Here's how the part is built. I have some questions about the finished solid (model axes, mm). Face numbers are marked on the shaded views. A direction names the side the tool comes from. Give positions to 0.01 mm unless a question says otherwise; leave off trailing zeros. Loops run counter-clockwise (first coordinate to the right, second up) from the corner with the lowest first, then second, coordinate; pieces in that order, holes last.
Q1. Suppose I cut it at C-C (z = 7). List the corners of the cut face in (x, y) for me.
Q2. Suppose I cut it at D-D (x = 0). List the corners of the cut face in (y, z) for me, and give its area (3 significant figures).
Q3. Suppose I cut it at B-B (x = 5). List the corners of the cut face in (y, z) for me, and give its area (3 significant figures).
Q4. Thinking about a two-plate mould opening in Z: for the marked faces 3, 4 and 5, which applies, pulls with the +Z half, pulls with the -Z half, needs draft (parallel to the pull), parting line crosses it, or undercut?
Q5. Suppose I cut it at A-A (z = 2). List the corners of the cut face in (x, y) for me.
Q6. I need wall thicknesses on probe 1 along X at (y, z) = (27.05, 0); probe 2 along Z at (x, y) = (6, 15.25); probe 3 along Y at (x, z) = (-2.5, 4.75). Which ranges of each line are inside material? Lowest first, please.
Q7. For the marked faces 1 and 2, which set-ups out of +Z, -Z, +X, -X, +Y, -Y let a thin tool reach every point of the face, with its end or its side?
```python
from build123d import *

# Parameters (mm, degrees)
SKETCH1_W           = 22
SKETCH1_H           = 28
BOSS_EXTRUDE1_DEPTH = 5
SKETCH2_W           = 22
SKETCH2_H           = 5
BOSS_EXTRUDE2_DEPTH = 20
SKETCH3_W           = 22
SKETCH3_H           = 28
BOSS_EXTRUDE3_DEPTH = 5
SKETCH4_R           = 1.55
CUT_EXTRUDE1_DEPTH  = 30
SKETCH5_W           = 22
SKETCH5_H           = 20
CUT_EXTRUDE2_DEPTH  = 1.5
SKETCH6_W           = 22
SKETCH6_H           = 20
CUT_EXTRUDE3_DEPTH  = 1.5


with BuildPart() as part:
    # Sketch1 → Boss-Extrude1 (new body)
    with BuildSketch(Plane(origin=(0, 0, 0), x_dir=(1, 0, 0), z_dir=(0, 1, 0))):
        Rectangle(SKETCH1_W, SKETCH1_H)
    extrude(amount=BOSS_EXTRUDE1_DEPTH)

    # Sketch2 → Boss-Extrude2 (add)
    with BuildSketch(Plane(origin=(0, 5, 0), x_dir=(1, 0, 0), z_dir=(0, 1, 0))):
        with Locations((0, -11.5)):
            Rectangle(SKETCH2_W, SKETCH2_H)
        with Locations((0, 11.5)):
            Rectangle(SKETCH2_W, SKETCH2_H)
    extrude(amount=BOSS_EXTRUDE2_DEPTH)

    # Sketch3 → Boss-Extrude3 (add)
    with BuildSketch(Plane(origin=(0, 25, 0), x_dir=(1, 0, 0), z_dir=(0, 1, 0))):
        Rectangle(SKETCH3_W, SKETCH3_H)
    extrude(amount=BOSS_EXTRUDE3_DEPTH)

    # Sketch4 → Cut-Extrude1 (cut)
    with BuildSketch(Plane(origin=(0, 30, 0), x_dir=(1, 0, 0), z_dir=(0, 1, 0))):
        with Locations(Location((0, 7, 0), (0, 0, 270))):
            Circle(SKETCH4_R)
        with Locations(Location((7, 0, 0), (0, 0, 270))):
            Circle(SKETCH4_R)
        with Locations(Location((0, -7, 0), (0, 0, 270))):
            Circle(SKETCH4_R)
        with Locations(Location((-7, 0, 0), (0, 0, 270))):
            Circle(SKETCH4_R)
    extrude(amount=-CUT_EXTRUDE1_DEPTH, mode=Mode.SUBTRACT)

    # Sketch5 → Cut-Extrude2 (cut)
    with BuildSketch(Plane.XY.offset(-9)):
        with Locations((0, 15)):
            Rectangle(SKETCH5_W, SKETCH5_H)
    extrude(amount=-CUT_EXTRUDE2_DEPTH, mode=Mode.SUBTRACT)

    # Sketch6 → Cut-Extrude3 (cut)
    with BuildSketch(Plane(origin=(0, 0, 9), x_dir=(-1, 0, 0), z_dir=(0, 0, -1))):
        with Locations((0, 15)):
            Rectangle(SKETCH6_W, SKETCH6_H)
    extrude(amount=-CUT_EXTRUDE3_DEPTH, mode=Mode.SUBTRACT)


solid = part.part
```
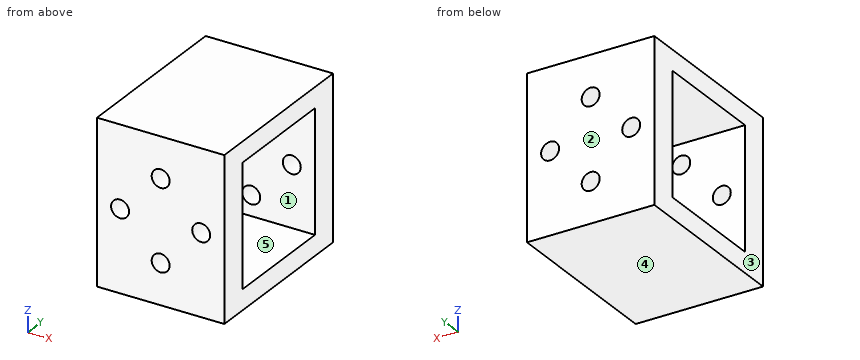
Solutions:
1. outline: (-11, 0) - (-1.55, 0) - (-1.55, 5) - (-11, 5) - close; (-11, 25) - (-1.55, 25) - (-1.55, 30) - (-11, 30) - close; (1.55, 0) - (11, 0) - (11, 5) - (1.55, 5) - close; (1.55, 25) - (11, 25) - (11, 30) - (1.55, 30) - close
2. outline: (0, -14) - (30, -14) - (30, -8.55) - (25, -8.55) - (25, -10.5) - (5, -10.5) - (5, -8.55) - (0, -8.55) - close; (0, -5.45) - (5, -5.45) - (5, 5.45) - (0, 5.45) - close; (0, 8.55) - (5, 8.55) - (5, 10.5) - (25, 10.5) - (25, 8.55) - (30, 8.55) - (30, 14) - (0, 14) - close; (25, -5.45) - (30, -5.45) - (30, 5.45) - (25, 5.45) - close
2. area: 358 mm2
3. outline: (0, -14) - (30, -14) - (30, 14) - (0, 14) - close; hole (5, -10.5) - (25, -10.5) - (25, 10.5) - (5, 10.5) - close
3. area: 420 mm2
4. face 3: needs draft
4. face 4: pulls with the -Z half
4. face 5: undercut
5. outline: (-11, 0) - (11, 0) - (11, 5) - (-11, 5) - close; (-11, 25) - (11, 25) - (11, 30) - (-11, 30) - close
6. probe 1: x = -11 to -8.55, -5.45 to 5.45, 8.55 to 11
6. probe 2: z = -14 to -10.5, 10.5 to 14
6. probe 3: y = 0 to 5, 25 to 30
7. face 1: +X, -X
7. face 2: +Z, -Z, +X, -X, +Y
